from build123d import *

# Parameters (mm, degrees)
SKETCH1_R                          = 63.373
BOSS_EXTRUDE1_DEPTH                = 1.5875
F_1_4_0_25_DIAMETER_HOLE1_D        = 6.35
F_5_16_0_3125_DIAMETER_HOLE1_D     = 7.9375
F_5_16_0_3125_DIAMETER_HOLE1_DEPTH = 3.302


with BuildPart() as part:
    # Sketch1 → Boss-Extrude1 (new body, symmetric)
    with BuildSketch(Plane.XY):
        Circle(SKETCH1_R)
    extrude(amount=BOSS_EXTRUDE1_DEPTH, both=True)

    # 1/4 (0.25) Diameter Hole1 (through all)
    with Locations(Plane.XY.offset(1.5875)):
        with Locations((-47.625, 0), (47.625, 0)):
            Hole(F_1_4_0_25_DIAMETER_HOLE1_D / 2)

    # 5/16 (0.3125) Diameter Hole1
    with Locations(Plane.XY.offset(1.5875)):
        with Locations((0, 0)):
            Hole(F_5_16_0_3125_DIAMETER_HOLE1_D / 2, depth=F_5_16_0_3125_DIAMETER_HOLE1_DEPTH)


solid = part.part
Read the model definition and answer for the solid it produces. Units are mm, in the model's axes. Coordinates: 2 decimals unless noted, no trailing zeros. Order: outer loops, then holes, each group sorted by start corner. A loop starts at its lowest first (then second) coordinate and runs counter-clockwise, first axis right, second up. Notation, with made-up numbers: (81, 79.25) - (114, 79.25) arc R24 cw to (114, 103.25) - close; hole circle Ø10 at (-32, 89). An arc over 180 degrees is marked (long way). Use one line per item in the form item = value.
(1) Given pin 1 Ø1 at (y, z) = (20.5, -0.5) entering from +X, flat-ended and moving along its own axis, determine where the tip first touches the part or whether it passes through.
Computed values:
pin_1 = 60.13
(2) Section C-C, the plane z = 0.75 is taken. Give the number of separate pieces and of enclosed holes in the cut face, then the cut area to 3 significant figures.
Computed values:
separate_pieces = 1
enclosed_holes = 3
area = 12,500 mm²
(3) Section B-B, the plane x = 0 is taken. Give the vertices of the cut face in (y, z).
Computed values:
outline = (-63.37, -1.59) - (-3.97, -1.59) - (-3.97, 1.59) - (-63.37, 1.59) - close; (3.97, -1.59) - (63.37, -1.59) - (63.37, 1.59) - (3.97, 1.59) - close
(4) For a pull along Y with two mould halves and no side action, classify faces 1 (the face through (13, 1, 1.588)), 2 (the face through (-46.71, 42.83, 0.02)), 3 (the face through (44.597, 0.954, -0.022)) as pulls with the +Y half, pulls with the -Y half, needs draft (parallel to the pull), parting line crosses it, or undercut.
Computed values:
face_1 = needs draft
face_2 = parting line crosses it
face_3 = undercut
(5) Section A-A, the plane y = 0 is taken. Give the vertices of the cut face in (x, z), then the cut area to 3 significant figures.
Computed values:
outline = (-63.37, -1.59) - (-50.8, -1.59) - (-50.8, 1.59) - (-63.37, 1.59) - close; (-44.45, -1.59) - (-3.97, -1.59) - (-3.97, 1.59) - (-44.45, 1.59) - close; (3.97, -1.59) - (44.45, -1.59) - (44.45, 1.59) - (3.97, 1.59) - close; (50.8, -1.59) - (63.37, -1.59) - (63.37, 1.59) - (50.8, 1.59) - close
area = 337 mm²
(6) Straight lines are drawn through the part: L1, parallel to Y at x = 0, z = -0.25; L2, parallel to Y at x = -50, z = 0.95; L3, parallel to Y at x = 28.5, z = -1.4. For each, find the intervals that lie inside material, in ascending order.
Computed values:
L1 = -63.37 to -3.97, 3.97 to 63.37
L2 = -38.94 to -2.11, 2.11 to 38.94
L3 = -56.6 to 56.6
(7) Section D-D, the plane x = -14.5 is taken. Give the vertices of the cut face in (y, z), then the cut area to 3 significant figures.
Computed values:
outline = (-61.69, -1.59) - (61.69, -1.59) - (61.69, 1.59) - (-61.69, 1.59) - close
area = 392 mm²
